Input: part model. Units: mm. Frame: model coordinates. Face numbers are marked on the shaded views. Give positions to 0.01 mm unless a question says otherwise; leave off trailing zeros. Order: outer loops, then holes, each group sorted by start corner. A loop starts at its lowest first (then second) coordinate and runs counter-clockwise, first axis right, second up.
```python
from build123d import *

# Parameters (mm, degrees)
SKETCH1_R                = 1.55
BOSS_EXTRUDE1_DEPTH      = 10.3
BOSS_EXTRUDE2_DEPTH      = 1
BOSS_EXTRUDE2_DEPTH_BACK = 1


with BuildPart() as part:
    # Sketch1 → Boss-Extrude1 (new body)
    with BuildSketch(Plane.XY):
        with BuildLine():
            Line((2, 0), (25.8, 0))
            ThreePointArc((25.8, 0), (27.214213562, 0.585786438), (27.8, 2))
            Line((27.8, 2), (27.8, 13.9))
            ThreePointArc((27.8, 13.9), (27.214213562, 15.314213562), (25.8, 15.9))
            Line((25.8, 15.9), (2, 15.9))
            ThreePointArc((2, 15.9), (0.585786438, 15.314213562), (0, 13.9))
            Line((0, 13.9), (0, 2))
            ThreePointArc((0, 2), (0.585786438, 0.585786438), (2, 0))
        make_face()
        with Locations(Location((2.8, 2.8, 0), (0, 0, 180))):
            Circle(SKETCH1_R, mode=Mode.SUBTRACT)
        with Locations(Location((25, 13.1, 0), (0, 0, 180))):
            Circle(SKETCH1_R, mode=Mode.SUBTRACT)
    extrude(amount=BOSS_EXTRUDE1_DEPTH)

    # Sketch2 → Boss-Extrude2 (add, two sides: drawn at the far end of the back side and taken through both)
    with BuildSketch(Plane.XY.offset(5.15).offset(-BOSS_EXTRUDE2_DEPTH_BACK)):
        with BuildLine():
            Line((6.55, 18.4), (6.55, 16.9))
            Line((6.55, 16.9), (7.05, 16.9))
            Line((7.05, 16.9), (19.1, 16.9))
            Line((19.1, 16.9), (19.1, 15.9))
            Line((19.1, 15.9), (19.6, 15.9))
            Line((19.6, 15.9), (19.6, 17.4))
            Line((19.6, 17.4), (7.05, 17.4))
            Line((7.05, 17.4), (7.05, 18.4))
            ThreePointArc((7.05, 18.4), (6.8, 20.773669459), (6.55, 18.4))
        make_face()
    extrude(amount=BOSS_EXTRUDE2_DEPTH + BOSS_EXTRUDE2_DEPTH_BACK)


solid = part.part
```
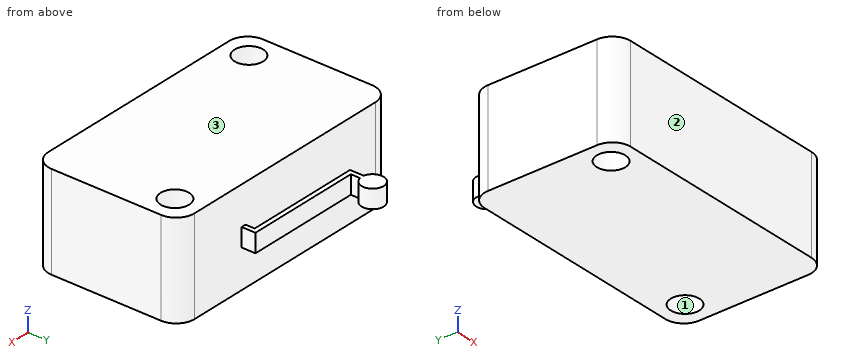
1) Cut plane B-B (z = 7.5). Return the cut outline in (x, y).
2) Line query: probe 1 along X at (y, z) = (13.1, 6); probe 2 along Y at (x, z) = (25, 4.5); probe 3 along Y at (x, z) = (2.8, 6.5). Output: solid intervals per line, ascending.
3) First-contact query: P1, Ø1.6, axis at y = 17.5, z = 5, coming from the -X side; P2, Ø4, axis at x = 19, z = 1.5, coming from the +Y side; P3, Ø1, axis at x = 18, y = 17, coming from the -Z side; P4, Ø4, axis at x = 3, z = 6.5, coming from the -Y side. Flat tips, straight axial feed; report the tip coordinate or a pass-through.
4) Cut plane D-D (z = 5.75). Return the cut outline in (x, y), then the cut area to 3 significant figures.
5) Cut plane A-A (y = 2.8). Return the cut outline in (x, z).
6) Cut plane C-C (x = 25). Return the cut outline in (y, z).
7) Pull-direction query (Y, two-part tool) for the marked faces 1, 2 and 3; classes: pulls with the +Y half, pulls with the -Y half, needs draft (parallel to the pull), parting line crosses it, or undercut.
Geometry says:
1. outline: (0, 2) arc R2 ccw to (2, 0) - (25.8, 0) arc R2 ccw to (27.8, 2) - (27.8, 13.9) arc R2 ccw to (25.8, 15.9) - (2, 15.9) arc R2 ccw to (0, 13.9) - close; hole circle Ø3.1 at (2.8, 2.8); hole circle Ø3.1 at (25, 13.1)
2. probe 1: x = 0 to 23.45, 26.55 to 27.8
2. probe 2: y = 0 to 11.55, 14.65 to 15.9
2. probe 3: y = 0 to 1.25, 4.35 to 15.9
3. P1: stops at x = 6.55
3. P2: stops at y = 15.9
3. P3: stops at z = 4.15
3. P4: stops at y = 0
4. outline: (0, 2) arc R2 ccw to (2, 0) - (25.8, 0) arc R2 ccw to (27.8, 2) - (27.8, 13.9) arc R2 ccw to (25.8, 15.9) - (19.6, 15.9) - (19.6, 17.4) - (7.05, 17.4) - (7.05, 18.4) arc R1.2 ccw (long way) to (6.55, 18.4) - (6.55, 16.9) - (19.1, 16.9) - (19.1, 15.9) - (2, 15.9) arc R2 ccw to (0, 13.9) - close; hole circle Ø3.1 at (2.8, 2.8); hole circle Ø3.1 at (25, 13.1)
4. area: 436 mm2
5. outline: (0, 0) - (1.25, 0) - (1.25, 10.3) - (0, 10.3) - close; (4.35, 0) - (27.8, 0) - (27.8, 10.3) - (4.35, 10.3) - close
6. outline: (0, 0) - (11.55, 0) - (11.55, 10.3) - (0, 10.3) - close; (14.65, 0) - (15.9, 0) - (15.9, 10.3) - (14.65, 10.3) - close
7. face 1: undercut
7. face 2: pulls with the -Y half
7. face 3: needs draft
